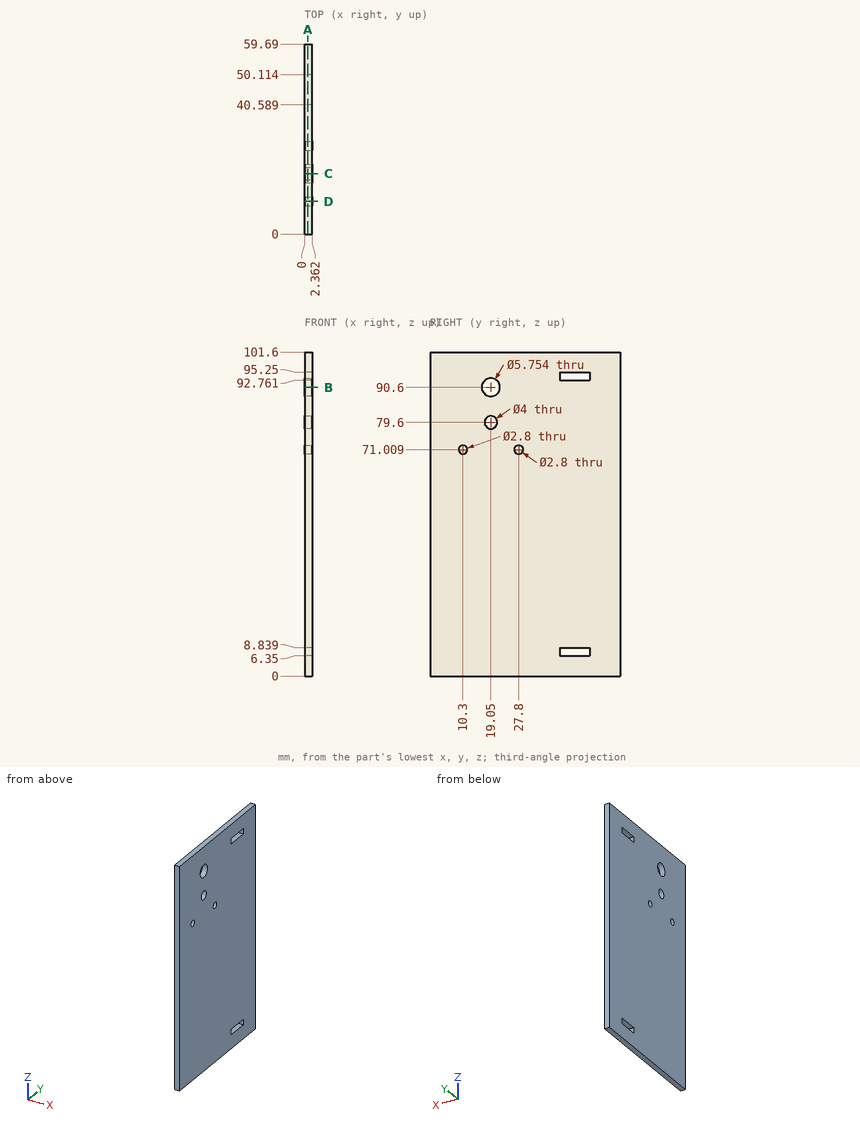
The drawing under review shows one solid part. Ordinate dimensions are in mm from its lowest x, y, z. Give positions to 0.01 mm unless a question says otherwise; leave off trailing zeros. Write each loop counter-clockwise with the first axis right and the second up, starting at its lowest first coordinate (ties: lowest second). Pieces come first, ordered by that corner, then holes. Notation, with made-up numbers: (42.5, 46.25) - (88.5, 46.25) arc R15 cw to (88.5, 54.25) - close; hole circle Ø3 at (0.5, 0). An arc over 180 degrees is marked (long way). Answer in a Markdown table with one row per item. Add a question column.
1. We need section B-B on z = 90.6. Write out the cut boundary in (x, y).
2. We need section D-D on y = 10.3. Write out the cut boundary in (x, z).
3. We need section C-C on y = 19.05. Write out the cut boundary in (x, z), then the cut area to 3 significant figures.
4. We need section A-A on x = 1. Write out the cut boundary in (y, z), then the cut area to 3 significant figures.
5. Wall thickness on line 1 along Y through (x, z) = (0.9, 71); line 2 along Z through (x, y) = (0.35, 44); line 3 along Y through (x, z) = (0.95, 90.6): over which ranges is each line inside the solid? List them lowest first. Write a range as [from, to].
Ans:
| question | item | result |
|---|---|---|
| 1 | outline | (0, 0) - (2.36, 0) - (2.36, 16.17) - (0, 16.17) - close; (0, 21.93) - (2.36, 21.93) - (2.36, 59.69) - (0, 59.69) - close |
| 2 | outline | (0, 0) - (2.36, 0) - (2.36, 69.61) - (0, 69.61) - close; (0, 72.41) - (2.36, 72.41) - (2.36, 101.6) - (0, 101.6) - close |
| 3 | outline | (0, 0) - (2.36, 0) - (2.36, 77.6) - (0, 77.6) - close; (0, 81.6) - (2.36, 81.6) - (2.36, 87.72) - (0, 87.72) - close; (0, 93.48) - (2.36, 93.48) - (2.36, 101.6) - (0, 101.6) - close |
| 3 | area | 217 mm^2 |
| 4 | outline | (0, 0) - (59.69, 0) - (59.69, 101.6) - (0, 101.6) - close; hole circle Ø2.8 at (10.3, 71.01); hole circle Ø5.75 at (19.05, 90.6); hole circle Ø4 at (19.05, 79.6); hole circle Ø2.8 at (27.8, 71.01); hole (40.59, 6.35) - (50.11, 6.35) - (50.11, 8.84) - (40.59, 8.84) - close; hole (40.59, 92.76) - (50.11, 92.76) - (50.11, 95.25) - (40.59, 95.25) - close |
| 4 | area | 5,970 mm^2 |
| 5 | line 1 | y = [0, 8.9], [11.7, 26.4], [29.2, 59.69] |
| 5 | line 2 | z = [0, 6.35], [8.84, 92.76], [95.25, 101.6] |
| 5 | line 3 | y = [0, 16.17], [21.93, 59.69] |
